Read the model definition and answer for the solid it produces. Units are mm, in the model's axes. A direction names the side the tool comes from. Give positions to 0.01 mm unless a question says otherwise; leave off trailing zeros. Write each loop counter-clockwise with the first axis right and the second up, starting at its lowest first coordinate (ties: lowest second). Pieces come first, ordered by that corner, then holes. Notation, with made-up numbers: (15, 59) -> (19, 59) arc R17 cw to (19, 66) -> close; hole circle Ø6 at (19, 30). An arc over 180 degrees is marked (long way). Put each result on its own line as item: value. Start each with the question number.
from build123d import *

# Parameters (mm, degrees)
SKETCH_1_W          = 15.8
SKETCH_1_H          = 15.8
EXTRUDE_1_DEPTH     = 9.6
SKETCH_2_R          = 2.4
EXTRUDE_2_DEPTH     = 1.7
SKETCH_3_R          = 2.5
CUT_EXTRUDE_2_DEPTH = 1.8


with BuildPart() as part:
    # Эскиз1 → Бобышка-Вытянуть1 (new body)
    with BuildSketch(Plane(origin=(0, 0, 0), x_dir=(1, 0, 0), z_dir=(0, 1, 0))):
        with Locations((7.9, 7.9)):
            Rectangle(SKETCH_1_W, SKETCH_1_H)
    extrude(amount=EXTRUDE_1_DEPTH)

    # Эскиз2 → Бобышка-Вытянуть2 (add)
    with BuildSketch(Plane(origin=(0, 9.6, 0), x_dir=(1, 0, 0), z_dir=(0, 1, 0))):
        with Locations((3.9, 11.9)):
            Circle(SKETCH_2_R)
        with Locations((11.9, 11.9)):
            Circle(SKETCH_2_R)
        with Locations((11.9, 3.9)):
            Circle(SKETCH_2_R)
        with Locations((3.9, 3.9)):
            Circle(SKETCH_2_R)
    extrude(amount=EXTRUDE_2_DEPTH)

    # Эскиз3 → Вырез-Вытянуть2 (cut)
    with BuildSketch(Plane.XZ):
        with Locations((11.9, -3.9)):
            Circle(SKETCH_3_R)
        with Locations((3.9, -3.9)):
            Circle(SKETCH_3_R)
        with Locations((3.9, -11.9)):
            Circle(SKETCH_3_R)
        with Locations((11.9, -11.9)):
            Circle(SKETCH_3_R)
    extrude(amount=-CUT_EXTRUDE_2_DEPTH, mode=Mode.SUBTRACT)


solid = part.part
1) Straight lines are drawn through the part: line 1 (Z direction, x = 3.9, y = 0.5); line 2 (X direction, y = 1.5, z = -9.75); line 3 (Z direction, x = 13.5, y = 0.75). For each, find the intervals that lie inside material, in ascending order. Write a range as [from, to].
2) A cutting plane is placed at D-D on x = 14.75. Give the vertices of the cut face in (y, z), and give its area (3 significant figures).
3) Each of these flat-tipped pins is pushed along its axis until it touches: pin 1 Ø1.5 at (x, z) = (5, -5) entering from -Y; pin 2 Ø1 at (x, z) = (7.5, -7) entering from +Y. Where does it stop, or does it pass through?
4) A cutting plane is placed at A-A on y = 1.25. Give the vertices of the cut face in (x, z), and give its area (3 significant figures).
5) A cutting plane is placed at B-B on x = 11.9. Give the vertices of the cut face in (y, z).
6) For a pull along X with two mould halves and no side action, classify faces 1 (the face through (4, 11.3, -12)), 2 (the face through (8, 9.6, -8)), 3 (the face through (0, 5, -8)) as pulls with the +X half, pulls with the -X half, needs draft (parallel to the pull), parting line crosses it, or undercut.
7) For faces 4 (the face through (8, 5, -15.8)), 5 (the face through (4, 1.8, -4)), 6 (the face through (5.01, 10.44, -1.77)), determine the directions among +Z, -Z, +X, -X, +Y, -Y from which every point of the face is accessible in a straight line to the end or side of a thin tool.
8) A cutting plane is placed at C-C on z = -3.9. Give the vertices of the cut face in (x, y).
Results found:
1. line 1: z = [-15.8, -14.4], [-9.4, -6.4], [-1.4, 0]
1. line 2: x = [0, 2.62], [5.18, 10.62], [13.18, 15.8]
1. line 3: z = [-15.8, -13.82], [-9.98, -5.82], [-1.98, 0]
2. outline: (0, -15.8) -> (9.6, -15.8) -> (9.6, 0) -> (0, 0) -> close
2. area: 152 mm²
3. pin 1: stops at y = 1.8
3. pin 2: stops at y = 9.6
4. outline: (0, -15.8) -> (15.8, -15.8) -> (15.8, 0) -> (0, 0) -> close; hole circle Ø5 at (3.9, -11.9); hole circle Ø5 at (3.9, -3.9); hole circle Ø5 at (11.9, -11.9); hole circle Ø5 at (11.9, -3.9)
4. area: 171 mm²
5. outline: (0, -15.8) -> (9.6, -15.8) -> (9.6, -14.3) -> (11.3, -14.3) -> (11.3, -9.5) -> (9.6, -9.5) -> (9.6, -6.3) -> (11.3, -6.3) -> (11.3, -1.5) -> (9.6, -1.5) -> (9.6, 0) -> (0, 0) -> (0, -1.4) -> (1.8, -1.4) -> (1.8, -6.4) -> (0, -6.4) -> (0, -9.4) -> (1.8, -9.4) -> (1.8, -14.4) -> (0, -14.4) -> close
6. face 1: needs draft
6. face 2: undercut
6. face 3: pulls with the -X half
7. face 4: -Z, +X, -X, +Y, -Y
7. face 5: -Y
7. face 6: +Y
8. outline: (0, 0) -> (1.4, 0) -> (1.4, 1.8) -> (6.4, 1.8) -> (6.4, 0) -> (9.4, 0) -> (9.4, 1.8) -> (14.4, 1.8) -> (14.4, 0) -> (15.8, 0) -> (15.8, 9.6) -> (14.3, 9.6) -> (14.3, 11.3) -> (9.5, 11.3) -> (9.5, 9.6) -> (6.3, 9.6) -> (6.3, 11.3) -> (1.5, 11.3) -> (1.5, 9.6) -> (0, 9.6) -> close
